Autodesk Inventor part; units mm, degrees
ref_plane "Work Plane1" through (0, 0, 0) normal (1, 0, 0) x (0, 1, 0)
ref_plane "XZ Plane" through (0, 0, 0) normal (0, 1, 0) x (-1, 0, 0)
ref_plane "XY Plane" through (0, 0, 0) normal (0, 0, 1) x (1, 0, 0)
sketch "Sketch1" plane through (0, 0, 0) normal (0, 1, 0) x (-1, 0, 0)
  circle A0 centre (0, 0) radius 87
  line L0 (10.5, 33.25) -> (-10.5, 33.25)
  line L1 (-10.5, 33.25) -> (-10.5, -33.25)
  line L2 (-10.5, -33.25) -> (10.5, -33.25)
  line L3 (10.5, -33.25) -> (10.5, 33.25)
  line L4 (10.5, 33.25) -> (-10.5, -33.25) construction
  line L5 (-10.5, 33.25) -> (10.5, -33.25) construction
  dimension "d0" = 174
  dimension "d1" = 21
  dimension "d2" = 66.5
ref_plane "Work Plane1" through (0, 0, 0) normal (1, 0, 0) x (0, 1, 0)
extrude "Extrusion2" add sketch "Sketch1" along normal blind 25.4
sketch "Sketch3" plane through (0, 25.4, 0) normal (0, 1, 0) x (1, 0, 0)
  circle A0 centre (0, 0) radius 86
  dimension "d63" = 172
hole "Hole2" at (0, 25.4, 0) direction (0, -1, 0) diameter 172 depth 23.4
properties part number "Bottom Cap"
Work out the finished part from the listing and answer in its coordinate system (mm). A direction names the side the tool comes from. Give positions to 0.01 mm unless a question says otherwise; leave off trailing zeros. Write each loop counter-clockwise with the first axis right and the second up, starting at its lowest first coordinate (ties: lowest second). Pieces come first, ordered by that corner, then holes. Notation, with made-up numbers: (60, 12) - (70, 12) arc R29 cw to (70, 47) - close; hole circle Ø4 at (82, -21). An arc over 180 degrees is marked (long way). Use one line per item in the form item = value.
1. A cutting plane is placed at A-A (x = 0). Write down the section's boundary in (y, z), and give its area (3 significant figures).
Filled in:
outline = (0, -87) - (25.4, -87) - (25.4, -86) - (2, -86) - (2, -33.25) - (0, -33.25) - close; (0, 33.25) - (2, 33.25) - (2, 86) - (25.4, 86) - (25.4, 87) - (0, 87) - close
area = 262 mm^2
2. Consider L1, parallel to Z at x = 0, y = 19.75; L2, parallel to X at y = 18.5, z = 70; L3, parallel to X at y = 15, z = 57.5. Determine where each line is inside the solid, lowest interval first.
Filled in:
L1 = -87 to -86, 86 to 87
L2 = -51.66 to -49.96, 49.96 to 51.66
L3 = -65.29 to -63.95, 63.95 to 65.29
3. A cutting plane is placed at B-B (z = -21). Write down the section's boundary in (x, y), and give its area (3 significant figures).
Filled in:
outline = (-84.43, 0) - (-10.5, 0) - (-10.5, 2) - (-83.4, 2) - (-83.4, 25.4) - (-84.43, 25.4) - close; (10.5, 0) - (84.43, 0) - (84.43, 25.4) - (83.4, 25.4) - (83.4, 2) - (10.5, 2) - close
area = 344 mm^2
4. For faces 1 (the face through (-85.268, 13.536, -11.195)), 2 (the face through (84, 25.4, 20)), determine the directions among +Z, -Z, +X, -X, +Y, -Y from which every point of the face is accessible in a straight line to the end or side of a thin tool.
Filled in:
face_1 = +Y
face_2 = +Z, -Z, +X, -X, +Y
5. A cutting plane is placed at C-C (y = 9). Write down the section's boundary in (x, z), and give its area (3 significant figures).
Filled in:
outline = circle Ø174 at (0, 0); hole circle Ø172 at (0, 0)
area = 543 mm^2
6. Each of these flat-tipped pins is pushed along its axis until it touches: pin 1 Ø1 at (x, y) = (3, 1) entering from -Z; pin 2 Ø8 at (x, y) = (-36.5, 21.5) entering from +Z; pin 3 Ø2 at (y, z) = (1, 12.5) entering from +X. Where does it stop, or does it pass through?
Filled in:
pin_1 = -86.96
pin_2 = 80.7
pin_3 = 86.24
7. A cutting plane is placed at D-D (x = 39). Write down the section's boundary in (y, z).
Filled in:
outline = (0, -77.77) - (25.4, -77.77) - (25.4, -76.65) - (2, -76.65) - (2, 76.65) - (25.4, 76.65) - (25.4, 77.77) - (0, 77.77) - close
8. Determine the mould class of faces 3 (the face through (-18, 0, 1)), 4 (the face through (18, 2, -1)), 5 (the face through (11.33, 12.52, -86.26)) for opening direction Z: released by +Z, released by -Z, zero draft, split by the parting line, or undercut.
Filled in:
face_3 = zero draft
face_4 = undercut
face_5 = split by the parting line
